Model file for the job. Use its own axes, mm. Coordinates: 2 decimals unless noted, no trailing zeros. Order: outer loops, then holes, each group sorted by start corner. A loop starts at its lowest first (then second) coordinate and runs counter-clockwise, first axis right, second up. Notation, with made-up numbers: (-0.5, 64.5) -> (45.5, 64.5) arc R29 ccw to (45.5, 94.5) -> close; hole circle Ø9 at (35.5, 8.25). An arc over 180 degrees is marked (long way). Write item = value, one per line. Start each with the question number.
Q1. Cut at B-B, the plane y = 52. List the corners of the cut face in (x, z).
Q2. Cut at A-A, the plane y = 87. List the corners of the cut face in (x, z).
Q3. Flat gauge pins, fed straight in: pin 1 (4 mm diameter, centred on y = 11.5, z = 6.5, fed in from -X); pin 2 (1 mm diameter, centred on x = 2.5, y = 86.5, fed in from -Z); pin 3 (0.6 mm diameter, centred on x = 1.5, y = 7.5, fed in from +Z). Where does each tip first touch, or does it go through?
Q4. Wall check: line 1 (Y direction, x = 2.2, z = 7); line 2 (Z direction, x = 2.3, y = 40); line 3 (Y direction, x = 0.3, z = -1.75). Give the ranges that are in metal, low to high. Write a range as from..to.
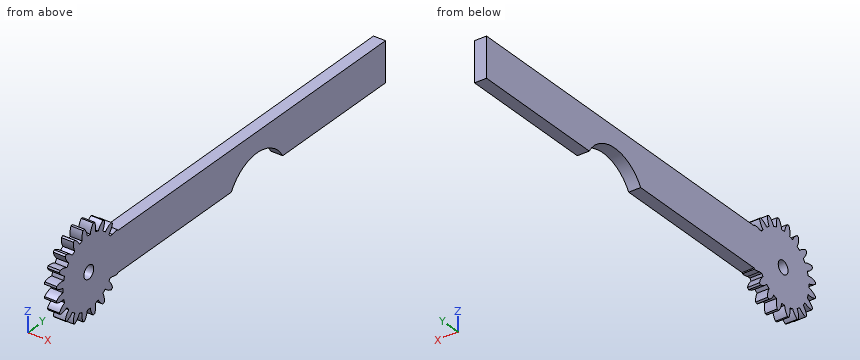
from build123d import *

# Parameters (mm, degrees)
BASPROSKE_W         = 3
BASPROSKE_H         = 11
TOOTHCUT_DEPTH      = 16.842979518
TEETHCUTS_COUNT     = 20
TEETHCUTS_ANGLE     = 342
BORSKE_R            = 2.5
BORE_DEPTH          = 50.0000508
SKETCH1_W           = 10
SKETCH1_H           = 100
BOSS_EXTRUDE1_DEPTH = 3
CUT_EXTRUDE1_DEPTH  = 3
CUT_EXTRUDE2_DEPTH  = 3
SKETCH6_R           = 2.5
SKETCH6_R_2         = 1.65
BOSS_EXTRUDE2_DEPTH = 3


with BuildPart() as part:
    # BasProSke → Base-Revolve (revolve)
    with BuildSketch(Plane(origin=(0, 0, 0), x_dir=(1, 0, 0), z_dir=(0, 1, 0)), mode=Mode.PRIVATE) as base_revolve_sk:
        with Locations((1.5, 5.5)):
            Rectangle(BASPROSKE_W, BASPROSKE_H)
    revolve(base_revolve_sk.sketch.rotate(Axis((-10, 0, 0), (1, 0, 0)), 180), axis=Axis((-10, 0, 0), (1, 0, 0)))

    # TooCutSke → ToothCut (cut, through all)
    with BuildSketch(Plane(origin=(0, 0, 0), x_dir=(0, 0, -1), z_dir=(1, 0, 0))):
        with BuildLine():
            ThreePointArc((0.499924007, 8.734705318), (0, 8.749), (-0.499924007, 8.734705318))
            ThreePointArc((-0.499924007, 8.734705318), (-0.824302243, 9.905497836), (-1.485192705, 10.924909509))
            ThreePointArc((-1.485192705, 10.924909509), (0, 11.0254), (1.485192705, 10.924909509))
            ThreePointArc((1.485192705, 10.924909509), (0.824302243, 9.905497836), (0.499924007, 8.734705318))
        make_face()
    toothcut = extrude(amount=TOOTHCUT_DEPTH, mode=Mode.SUBTRACT)

    # TeethCuts: ToothCut ×20 about axis
    teethcuts_axis = Axis((-10, 0, 0), (1, 0, 0))
    for i in range(1, TEETHCUTS_COUNT):
        add(toothcut.rotate(teethcuts_axis, i * TEETHCUTS_ANGLE / (TEETHCUTS_COUNT - 1)), mode=Mode.SUBTRACT)

    # BorSke → Bore (cut, symmetric)
    with BuildSketch(Plane(origin=(0, 0, 0), x_dir=(0, 0, -1), z_dir=(1, 0, 0))):
        with Locations(Location((0, 0, 0), (0, 0, 180))):
            Circle(BORSKE_R)
    extrude(amount=BORE_DEPTH, both=True, mode=Mode.SUBTRACT)

    # Sketch1 → Boss-Extrude1 (add)
    with BuildSketch(Plane(origin=(3, 0, 0), x_dir=(0, 0, -1), z_dir=(1, 0, 0))):
        with Locations((0, 50)):
            Rectangle(SKETCH1_W, SKETCH1_H)
    extrude(amount=-BOSS_EXTRUDE1_DEPTH)

    # Sketch4 → Cut-Extrude1 (cut)
    with BuildSketch(Plane(origin=(3, 0, 0), x_dir=(0, 0, -1), z_dir=(1, 0, 0))):
        with BuildLine():
            Line((5, 65.352905548), (5, 48.032397472))
            ThreePointArc((5, 48.032397472), (0, 56.69265151), (5, 65.352905548))
        make_face()
    extrude(amount=-CUT_EXTRUDE1_DEPTH, mode=Mode.SUBTRACT)

    # Sketch5 → Cut-Extrude2 (cut)
    with BuildSketch(Plane(origin=(3, 0, 0), x_dir=(0, 0, -1), z_dir=(1, 0, 0))):
        with BuildLine():
            Line((2.5, 0), (-2.5, 0))
            ThreePointArc((-2.5, 0), (0, 2.5), (2.5, 0))
        make_face()
    extrude(amount=-CUT_EXTRUDE2_DEPTH, mode=Mode.SUBTRACT)

    # Sketch6 → Boss-Extrude2 (add)
    with BuildSketch(Plane(origin=(3, 0, 0), x_dir=(0, 0, -1), z_dir=(1, 0, 0))):
        Circle(SKETCH6_R)
        Circle(SKETCH6_R_2, mode=Mode.SUBTRACT)
    extrude(amount=-BOSS_EXTRUDE2_DEPTH)


solid = part.part
Here are the results:
q1.outline = (0, -1.17) -> (3, -1.17) -> (3, 5) -> (0, 5) -> close
q2.outline = (0, -5) -> (3, -5) -> (3, 5) -> (0, 5) -> close
q3.pin_1 = 0
q3.pin_2 = -5
q3.pin_3 = 7.96
q4.line_1 = -7.78..-5.77, -5.25..5.25, 5.77..7.78
q4.line_2 = -5..5
q4.line_3 = -10.86..51.04, 62.34..100
